```python
from build123d import *

# Parameters (mm, degrees)
PAD_DEPTH               = 60
THICKNESS_T             = -2
SKETCH001_R             = 1.5
PAD001_DEPTH            = 57
SKETCH001_MIRRORED_2_R  = 1.5
PAD001_MIRRORED_2_DEPTH = 57
CHAMFER001_SIZE         = 3
CHAMFER003_SIZE         = 3


with BuildPart() as part:
    # Sketch → Pad (new body)
    with BuildSketch(Plane.XY):
        with BuildLine():
            Line((-82.5, 50), (-82.5, -50))
            ThreePointArc((-82.5, -50), (-81.035534, -53.535534), (-77.5, -55))
            Line((-77.5, -55), (77.5, -55))
            ThreePointArc((77.5, -55), (81.035534, -53.535534), (82.5, -50))
            Line((82.5, -50), (82.5, 50))
            ThreePointArc((82.5, 50), (81.035534, 53.535534), (77.5, 55))
            Line((77.5, 55), (-77.5, 55))
            ThreePointArc((-77.5, 55), (-81.035534, 53.535534), (-82.5, 50))
        make_face()
    extrude(amount=PAD_DEPTH)

    # Thickness
    thickness_openings = [part.faces().sort_by_distance(p)[0] for p in [
        (0, 0, 60),
    ]]
    offset(amount=THICKNESS_T, openings=thickness_openings)

    # Sketch001 → Pad001 (join)
    with BuildSketch(Plane.XY):
        with BuildLine():
            Line((-80.5, 53), (-73, 53))
            ThreePointArc((-80.5, 45.5), (-75.196699, 47.696699), (-73, 53))
            Line((-80.5, 53), (-80.5, 45.5))
        make_face()
        with Locations((-77.5, 50)):
            Circle(SKETCH001_R, mode=Mode.SUBTRACT)
    pad001 = extrude(amount=PAD001_DEPTH)

    # Sketch001 Mirrored 2 → Pad001 Mirrored 2 (add)
    with BuildSketch(Plane(origin=(0, 0, 0), x_dir=(-1, 0, 0), z_dir=(0, 0, -1))):
        with BuildLine():
            Line((-80.5, 53), (-73, 53))
            ThreePointArc((-80.5, 45.5), (-75.196699, 47.696699), (-73, 53))
            Line((-80.5, 53), (-80.5, 45.5))
        make_face()
        with Locations((-77.5, 50)):
            Circle(SKETCH001_MIRRORED_2_R, mode=Mode.SUBTRACT)
    pad001_mirrored_2 = extrude(amount=-PAD001_MIRRORED_2_DEPTH)

    # Mirrored001: Pad001, Pad001 Mirrored 2 across Sketch001 H_Axis
    add(pad001.mirror(Plane.ZX))
    add(pad001_mirrored_2.mirror(Plane.ZX))

    # Chamfer001
    chamfer001_edges = [part.edges().sort_by_distance(p)[0] for p in [
        (-75.196699, 47.696699, 2),
        (75.196699, 47.696699, 2),
        (75.196699, -47.696699, 2),
        (-75.196699, -47.696699, 2),
        (0, 53, 2),
        (-80.5, 0, 2),
        (0, -53, 2),
        (80.5, 0, 2),
    ]]
    chamfer(chamfer001_edges, length=CHAMFER001_SIZE)

    # Chamfer003
    chamfer003_edges = [part.edges().sort_by_distance(p)[0] for p in [
        (0, -55, 0),
    ]]
    chamfer(chamfer003_edges, length=CHAMFER003_SIZE)


solid = part.part
```
Could you check a few things on this model? Use its own coordinates, in mm. A direction names the side the tool comes from. Give positions to 0.01 mm unless a question says otherwise; leave off trailing zeros. Loops run counter-clockwise (first coordinate to the right, second up) from the corner with the lowest first, then second, coordinate; pieces in that order, holes last. Notation, with made-up numbers: (32, 63) - (55, 63) arc R19 ccw to (55, 97) - close; hole circle Ø2 at (57, 1.25). An arc over 180 degrees is marked (long way). Answer in a Markdown table with one row per item. Add a question column.
Q1. If we section it at C-C (x = 14.5): List the corners of the cut face in (y, z) for me, plus the area to 3 significant figures.
Q2. Please list where these lines run through material, in increasing order: L1, parallel to X at y = 0.5, z = 53; L2, parallel to Y at x = -29.5, z = 11.5; L3, parallel to Y at x = 77, z = 45. Write a range as from..to.
Q3. If we section it at B-B (y = -4): List the corners of the cut face in (x, z) for me, plus the area to 3 significant figures.
Q4. For pin 1 (1.5 mm diameter, centred on x = -77, y = -50, fed in from +Z); pin 2 (8.5 mm diameter, centred on x = -76.5, y = 48, fed in from +Z); pin 3 (3.5 mm diameter, centred on x = -77.5, y = -50, fed in from +Z), each with a flat end and sliding along its axis, tell me the tip position at first contact or that it passes through.
Q5. Which directions (+Z, -Z, +X, -X, +Y, -Y) give clear straight access to the entire face, cutting with the end or side of a thin tool? Please do faces 1 (the face through (-82.5, 1, 31)), 2 (the face through (1, 53, 32)).
Q6. If we section it at A-A (z = 32.5): List the corners of the cut face in (x, y) for me, plus the area to 3 significant figures.
Q7. We'd pull the mould along X, two halves only. Please class faces 3 (the face through (-81.07, -53.5, 31.1)), 4 (the face through (1, 55, 31)), 5 (the face through (-75.255, 47.639, 30.636)): +X half, -X half, draft (parallel to the pull), parting line (faces both ways), or undercut.
The answers:
| question | item | result |
|---|---|---|
| 1 | outline | (-55, 3) - (-52, 0) - (52, 0) - (55, 3) - (55, 60) - (53, 60) - (53, 5) - (50, 2) - (-50, 2) - (-53, 5) - (-53, 60) - (-55, 60) - close |
| 1 | area | 452 mm^2 |
| 2 | L1 | x = -82.5..-80.5, 80.5..82.5 |
| 2 | L2 | y = -55..-53, 53..55 |
| 2 | L3 | y = -55..-51.41, -48.59..-46.37, 46.37..48.59, 51.41..55 |
| 3 | outline | (-82.5, 3) - (-79.5, 0) - (79.5, 0) - (82.5, 3) - (82.5, 60) - (80.5, 60) - (80.5, 5) - (77.5, 2) - (-77.5, 2) - (-80.5, 5) - (-80.5, 60) - (-82.5, 60) - close |
| 3 | area | 562 mm^2 |
| 4 | pin 1 | stops at z = 2 |
| 4 | pin 2 | stops at z = 60 |
| 4 | pin 3 | stops at z = 57 |
| 5 | face 1 | +Z, -Z, -X, +Y, -Y |
| 5 | face 2 | +Z |
| 6 | outline | (-82.5, -50) arc R5 ccw to (-77.5, -55) - (77.5, -55) arc R5 ccw to (82.5, -50) - (82.5, 50) arc R5 ccw to (77.5, 55) - (-77.5, 55) arc R5 ccw to (-82.5, 50) - close; hole (-80.5, -45.5) arc R7.5 cw to (-73, -53) - (73, -53) arc R7.5 cw to (80.5, -45.5) - (80.5, 45.5) arc R7.5 cw to (73, 53) - (-73, 53) arc R7.5 cw to (-80.5, 45.5) - close; hole circle Ø3 at (-77.5, -50); hole circle Ø3 at (-77.5, 50); hole circle Ø3 at (77.5, -50); hole circle Ø3 at (77.5, 50) |
| 6 | area | 1,210 mm^2 |
| 7 | face 3 | -X half |
| 7 | face 4 | draft |
| 7 | face 5 | undercut |
